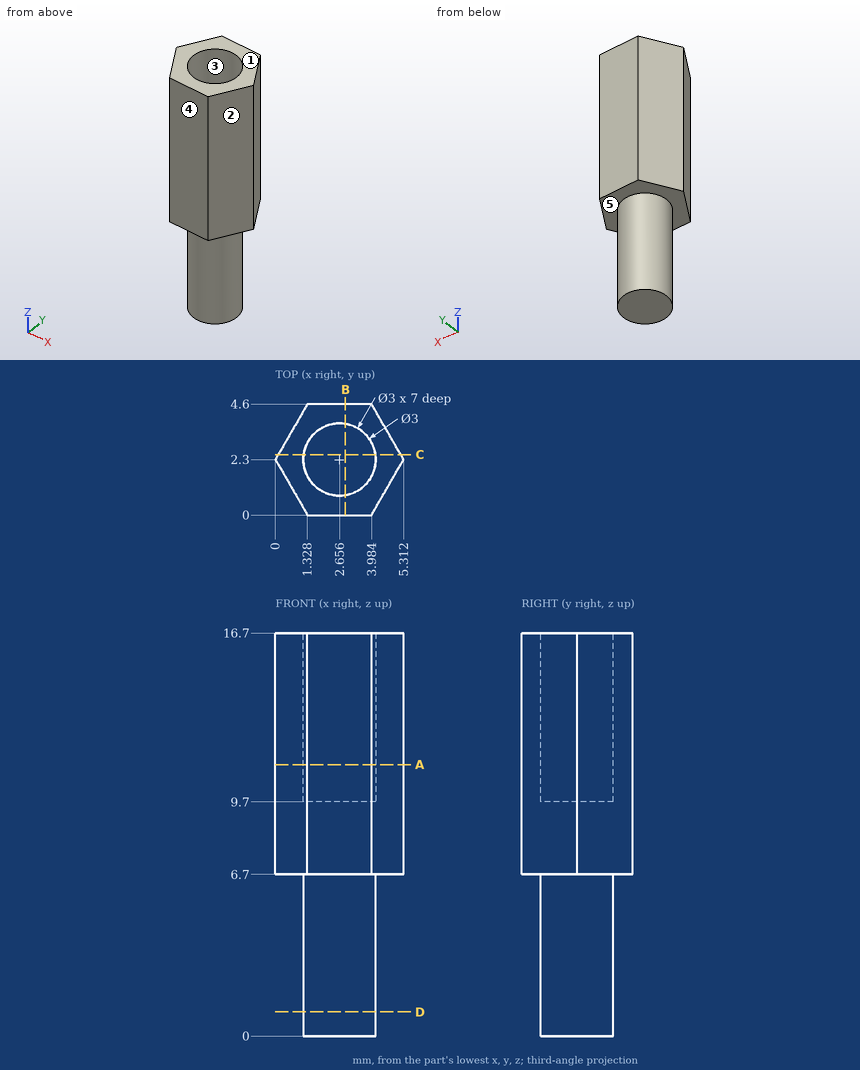
Here's the drawing with two shaded views (mm, measured from the low corner). I have some questions. A direction names the side the tool comes from. Round coordinates to 2 decimals unless told otherwise and drop trailing zeros. Loops run counter-clockwise (first coordinate to the right, second up) from the corner with the lowest first, then second, coordinate; pieces in that order, holes last. Notation, with made-up numbers: (5, 13) - (15, 13) arc R20 ccw to (15, 25) - close; hole circle Ø5 at (-15, -31). An arc over 180 degrees is marked (long way). Use CSV: the item, a comma, the result in double quotes. Start each with the question number.
1) For the marked faces 4 and 5, which set-ups out of +Z, -Z, +X, -X, +Y, -Y let a thin tool reach every point of the face, with its end or its side?
2) We'd pull the mould along Y, two halves only. Please class the marked faces 1, 2 and 3: released by +Y, released by -Y, zero draft, split by the parting line, or undercut.
3) If we section it at A-A on z = 11.25: Write out the boundary of the cut face in (x, y).
4) If we section it at C-C on y = 2.5: Write out the boundary of the cut face in (x, z) (1 decimal).
5) If we section it at D-D on z = 1: Write out the boundary of the cut face in (x, y).
6) For pin 1 Ø2.5 at (x, y) = (2.66, 2.3) entering from +Z, with a flat end and sliding along its axis, tell me the tip position at first contact or that it passes through.
7) If we section it at B-B on x = 2.9: Write out the boundary of the cut face in (y, z).
8) Please list where these lines run through material, in increasing order: probe 1 along Z at (x, y) = (2.1, 2.1); probe 2 along Z at (x, y) = (3.5, 0.3); probe 3 along Y at (x, z) = (2.4, 15). Write a range as [from, to].
Geometry results:
1,face 4,"+Z, -Z, +X, -X, -Y"
1,face 5,"-Z"
2,face 1,"zero draft"
2,face 2,"released by -Y"
2,face 3,"undercut"
3,outline,"(0, 2.3) - (1.33, 0) - (3.98, 0) - (5.31, 2.3) - (3.98, 4.6) - (1.33, 4.6) - close; hole circle Ø3 at (2.66, 2.3)"
4,outline,"(0.1, 6.7) - (1.2, 6.7) - (1.2, 0) - (4.1, 0) - (4.1, 6.7) - (5.2, 6.7) - (5.2, 16.7) - (4.1, 16.7) - (4.1, 9.7) - (1.2, 9.7) - (1.2, 16.7) - (0.1, 16.7) - close"
5,outline,"circle Ø3 at (2.66, 2.3)"
6,pin 1,"stops at z = 9.7"
7,outline,"(0, 6.7) - (0.82, 6.7) - (0.82, 0) - (3.78, 0) - (3.78, 6.7) - (4.6, 6.7) - (4.6, 16.7) - (3.78, 16.7) - (3.78, 9.7) - (0.82, 9.7) - (0.82, 16.7) - (0, 16.7) - close"
8,probe 1,"z = [0, 9.7]"
8,probe 2,"z = [6.7, 16.7]"
8,probe 3,"y = [0, 0.82], [3.78, 4.6]"
